Source: CAD feature listing. Evaluate the final solid. Frame: model axes, mm. Face numbers are marked on the shaded views. A direction names the side the tool comes from. Round coordinates to 2 decimals unless told otherwise and drop trailing zeros. Write each loop counter-clockwise with the first axis right and the second up, starting at its lowest first coordinate (ties: lowest second). Pieces come first, ordered by that corner, then holes.
Autodesk Inventor part; units mm, degrees
ref_plane "YZ Plane" through (0, 0, 0) normal (1, 0, 0) x (0, 1, 0)
ref_plane "XZ Plane" through (0, 0, 0) normal (0, 1, 0) x (-1, 0, 0)
ref_plane "XY Plane" through (0, 0, 0) normal (0, 0, 1) x (1, 0, 0)
sketch "Sketch1" plane through (0, 0, 0) normal (0, 0, 1) x (1, 0, 0)
  line L0 (17.9, -19.1) -> (17.9, 19.1)
  line L1 (15.9, 21.1) -> (-15.9, 21.1)
  line L2 (-17.9, 19.1) -> (-17.9, -19.1)
  line L3 (-15.9, -21.1) -> (-10.5924, -21.1)
  line L4 (17.9, -21.1) -> (-17.9, 21.1) construction
  line L5 (17.9, 21.1) -> (-17.9, -21.1) construction
  line L6 (-7.4, -17.4) -> (7.4, -17.4)
  line L7 (-7.4, -17.4) -> (-8.833, -20.051)
  line L8 (7.4, -17.4) -> (8.833, -20.051)
  line L9 (10.5924, -21.1) -> (15.9, -21.1)
  line L10 (-9.4, -21.1) -> (9.4, -21.1)
  arc A0 (-15.9, 21.1) -> (-17.9, 19.1) centre (-15.9, 19.1) ccw
  arc A1 (17.9, 19.1) -> (15.9, 21.1) centre (15.9, 19.1) ccw
  arc A2 (15.9, -21.1) -> (17.9, -19.1) centre (15.9, -19.1) ccw
  arc A3 (8.833, -20.051) -> (10.5924, -21.1) centre (10.5924, -19.1) ccw
  arc A4 (-10.5924, -21.1) -> (-8.833, -20.051) centre (-10.5924, -19.1) ccw
  arc A5 (-17.9, -19.1) -> (-15.9, -21.1) centre (-15.9, -19.1) ccw
  point P0 (0, 0)
  dimension "d0" = 35.8
  dimension "d1" = 42.2
  dimension "d2" = 38.5
  dimension "d3" = 10.5
  dimension "d4" = 10.5
  dimension "d5" = 8.5
  dimension "d6" = 8.5
  dimension "d7" = 2
extrude "Extrusion1" add sketch "Sketch1" along normal blind 1.8
sketch "Sketch2" plane through (0, 0, 1.8) normal (0, 0, 1) x (1, 0, 0)
  line L0 (-15.85, 15.1) -> (15.85, 15.1)
  line L1 (15.85, 15.1) -> (15.85, 17.6)
  line L2 (15.85, 17.6) -> (-15.85, 17.6)
  line L3 (-15.85, 17.6) -> (-15.85, 15.1)
  line L4 (-15.85, 15.1) -> (15.85, 17.6) construction
  line L5 (15.85, 15.1) -> (-15.85, 17.6) construction
  line L6 (15.9, 21.1) -> (-15.9, 21.1)
  point P0 (0, 0)
  point P1 (0, 16.35)
  point P2 (0, 16.35)
  point P3 (15.85, 16.35)
  point P4 (-15.85, 16.35)
  dimension "d10" = 2.5
  dimension "d11" = 6
  dimension "d12" = 31.7
extrude "Extrusion2" add sketch "Sketch2" along normal blind 1
fillet "Fillet1" radius 1 2 edges at (0, 17.6, 2.8) (0, 15.1, 2.8)
sketch "Sketch3" plane through (0, 0, 1.8) normal (0, 0, 1) x (1, 0, 0)
  line L0 (-12.9, 19.1) -> (12.9, 19.1)
  line L1 (13.9, 18.1) -> (13.9, -13.2)
  line L2 (12.9, -14.2) -> (-12.9, -14.2)
  line L3 (-13.9, -13.2) -> (-13.9, 18.1)
  line L4 (15.9, 21.1) -> (-15.9, 21.1)
  line L5 (-13.9, 2.9131) -> (-17.9, 2.9131)
  line L6 (-17.9, 19.1) -> (-17.9, -19.1)
  line L7 (13.9, 2.9131) -> (17.9, 2.9131)
  line L8 (17.9, -19.1) -> (17.9, 19.1)
  arc A0 (-12.9, 19.1) -> (-13.9, 18.1) centre (-12.9, 18.1) ccw
  arc A1 (13.9, 18.1) -> (12.9, 19.1) centre (12.9, 18.1) ccw
  arc A2 (12.9, -14.2) -> (13.9, -13.2) centre (12.9, -13.2) ccw
  arc A3 (-13.9, -13.2) -> (-12.9, -14.2) centre (-12.9, -13.2) ccw
  point P0 (0, 0)
  point P1 (13.9, -14.2)
  point P2 (13.9, 19.1)
  point P3 (-13.9, -14.2)
  dimension "d16" = 27.8
  dimension "d17" = 33.3
  dimension "d18" = 2
  dimension "d19" = 1
extrude "Extrusion3" add sketch "Sketch3" along normal blind 3.7
sketch "Sketch4" plane through (0, 0, 0) normal (0, 0, -1) x (-1, 0, 0)
  line L0 (-17.9, -19.1) -> (-17.9, 19.1)
  line L1 (17.9, 19.1) -> (17.9, -19.1)
  line L2 (-17.9, 6.6) -> (17.9, 6.6)
  line L3 (17.9, 6.6) -> (17.9, 4.1)
  line L4 (17.9, 4.1) -> (-17.9, 4.1)
  line L5 (-17.9, 4.1) -> (-17.9, 6.6)
  line L6 (-15.9, 21.1) -> (15.9, 21.1)
  point P0 (0, 0)
  dimension "d22" = 2.5
  dimension "d23" = 17
extrude "Extrusion4" add sketch "Sketch4" along normal blind 1
fillet "Fillet2" radius 1 2 edges at (0, 6.6, -1) (0, 4.1, -1)
sketch "Sketch5" plane through (0, 0, 0) normal (0, 0, -1) x (-1, 0, 0)
  line L0 (-14.8, 8.9) -> (14.8, 8.9)
  line L1 (15.8, 7.9) -> (15.8, -0.1)
  line L2 (14.8, -1.1) -> (-14.8, -1.1)
  line L3 (-15.8, -0.1) -> (-15.8, 7.9)
  line L4 (-15.9, 21.1) -> (15.9, 21.1)
  line L5 (-17.9, 6.6) -> (-17.9, 19.1)
  line L6 (17.9, 4.1) -> (17.9, -19.1)
  arc A0 (-15.8, -0.1) -> (-14.8, -1.1) centre (-14.8, -0.1) ccw
  arc A1 (-14.8, 8.9) -> (-15.8, 7.9) centre (-14.8, 7.9) ccw
  arc A2 (15.8, 7.9) -> (14.8, 8.9) centre (14.8, 7.9) ccw
  arc A3 (14.8, -1.1) -> (15.8, -0.1) centre (14.8, -0.1) ccw
  point P0 (0, 0)
  point P1 (0, 8.9)
  dimension "d27" = 22.2
  dimension "d28" = 2.1
  dimension "d29" = 10
  dimension "d30" = 2.1
  dimension "d31" = 1
extrude "Extrusion5" add sketch "Sketch5" along normal blind 26.3
sketch "Sketch6" plane through (0, 0, 0) normal (0, 0, -1) x (-1, 0, 0)
  line L0 (-5, 16.9799) -> (5, 16.9799)
  line L1 (5, 16.9799) -> (5, 8.9)
  line L2 (5, 8.9) -> (-5, 8.9)
  line L3 (-5, 8.9) -> (-5, 16.9799)
  line L4 (14.8, 8.9) -> (-14.8, 8.9)
  line L5 (5, 16.9799) -> (17.9, 16.9799)
  line L6 (17.9, 19.1) -> (17.9, 6.6)
  line L7 (-5, 16.9799) -> (-17.9, 16.9799)
  line L8 (-17.9, -19.1) -> (-17.9, 19.1)
  point P0 (0, 0)
  point P1 (-5, 12.94)
  dimension "d34" = 10
extrude "Extrusion6" cut sketch "Sketch6" against normal blind 4.5
sketch "Sketch7" plane through (-14.8, 8.9, -26.3) normal (0, 1, 0) x (1, 0, 0)
  line L0 (9.8, -30.8) -> (19.8, -30.8)
  line L1 (14.8, -30.8) -> (14.8, -11.8)
  line L2 (8.8, -11.8) -> (20.8, -11.8)
  line L3 (20.8, -11.8) -> (20.8, -10.8)
  line L4 (20.8, -10.8) -> (8.8, -10.8)
  line L5 (8.8, -10.8) -> (8.8, -11.8)
  line L6 (20.8, -11.8) -> (20.8, -26.3)
  line L7 (20.8, -26.3) -> (19.8, -26.3)
  line L8 (19.8, -26.3) -> (19.8, -11.8)
  line L9 (8.8, -11.8) -> (8.8, -26.3)
  line L10 (8.8, -26.3) -> (9.8, -26.3)
  line L11 (9.8, -26.3) -> (9.8, -11.8)
  point P0 (14.8, -26.3)
  dimension "d37" = 19
  dimension "d38" = 12
  dimension "d39" = 1
  dimension "d40" = 1
  dimension "d41" = 14.5
extrude "Extrusion7" add sketch "Sketch7" along normal blind 2
sketch "Sketch8" plane through (-14.8, 10.9, -26.3) normal (0, 1, 0) x (1, 0, 0)
  line L0 (9.8, -11.8) -> (19.8, -11.8)
  line L1 (20.8, -26.3) -> (20.8, -10.8)
  line L2 (19.8, -11.8) -> (20.8, -11.8)
  line L3 (20.8, -11.8) -> (20.8, -25.8)
  line L4 (20.8, -25.8) -> (19.8, -25.8)
  line L5 (19.8, -25.8) -> (19.8, -11.8)
  line L6 (9.8, -11.8) -> (9.8, -30.8)
  line L7 (8.8, -26.3) -> (8.8, -10.8)
  line L8 (9.8, -11.8) -> (8.8, -11.8)
  line L9 (8.8, -11.8) -> (8.8, -25.8)
  line L10 (8.8, -25.8) -> (9.8, -25.8)
  line L11 (9.8, -25.8) -> (9.8, -11.8)
  point P0 (14.8, -26.3)
  point P1 (9.8, -25.8)
  point P2 (9.8, -25.8)
extrude "Extrusion8" add sketch "Sketch8" along normal blind 2
sketch "Sketch9" plane through (5, 8.9, -14.5) normal (-1, 0, 0) x (0, 0, 1)
  line L0 (0, 2) -> (0, 4)
  line L1 (14, 0) -> (14, 4)
  line L2 (0, 4) -> (14, 4)
  line L3 (14, 4) -> (14, 2)
  line L4 (14, 2) -> (0, 2)
  line L5 (0, 2) -> (0, 4)
  point P0 (14.5, -8.9)
  point P1 (0, 2)
extrude "Extrusion9" add sketch "Sketch9" along normal blind 0.5
chamfer "Chamfer1" distance 2 angle 35 1 edges at (4.5, 12.9, -7.5) measured on face at (4.5, 11.5667, -5.1667)
mirror "Mirror1" about plane through (0, 0, 0) normal (1, 0, 0) of "Extrusion9", "Chamfer1"
sketch "Sketch10" plane through (0, 0, 4.5) normal (0, 0, -1) x (-1, 0, 0)
  line L0 (-4.5, 9.9) -> (4.5, 9.9)
  line L1 (5, 10.4) -> (5, 12.2)
  line L2 (4.5, 12.7) -> (-4.5, 12.7)
  line L3 (-5, 12.2) -> (-5, 10.4)
  line L4 (5, 8.9) -> (-5, 8.9)
  line L5 (-5, 8.9) -> (-5, 16.9799)
  arc A0 (-5, 10.4) -> (-4.5, 9.9) centre (-4.5, 10.4) ccw
  arc A1 (-4.5, 12.7) -> (-5, 12.2) centre (-4.5, 12.2) ccw
  arc A2 (5, 12.2) -> (4.5, 12.7) centre (4.5, 12.2) ccw
  arc A3 (4.5, 9.9) -> (5, 10.4) centre (4.5, 10.4) ccw
  point P0 (0, 0)
  point P1 (-5, 11.3)
  dimension "d51" = 1
  dimension "d52" = 10
  dimension "d53" = 0.5
  dimension "d54" = 2.8
extrude "Extrusion10" cut sketch "Sketch10" against normal blind 2
properties part number "PS2 USB C PD Mount"
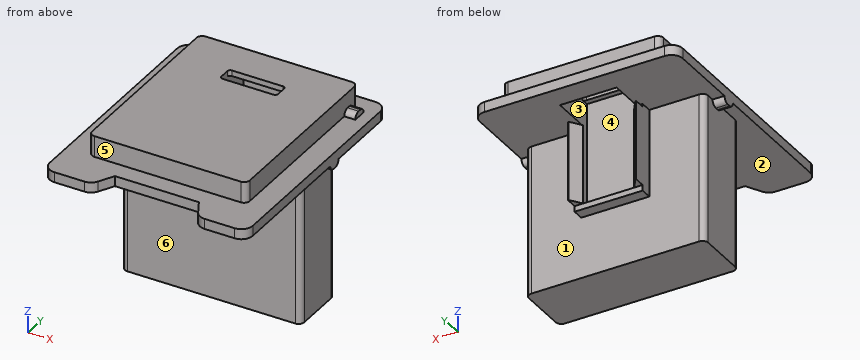
1) Section query A-A on x = -1.5. Return the cut outline in (y, z).
Taken from the geometry:
outline: (-17.4, 0) - (-1.1, 0) - (-1.1, -26.3) - (8.9, -26.3) - (8.9, -15.5) - (10.9, -15.5) - (10.9, -14.5) - (8.9, -14.5) - (8.9, 4.5) - (9.9, 4.5) - (9.9, 5.5) - (-14.2, 5.5) - (-14.2, 1.8) - (-17.4, 1.8) - close; (12.7, 4.5) - (16.98, 4.5) - (16.98, 0) - (21.1, 0) - (21.1, 1.8) - (19.1, 1.8) - (19.1, 5.5) - (12.7, 5.5) - close
2) Contact query for flat-ended pins moving along their axis: P1, Ø1.5, axis at x = 6, y = -6, coming from the -Z side; P2, Ø0.6, axis at x = 1.5, y = 10, coming from the -Z side; P3, Ø3, axis at x = -1.5, z = -9.5, coming from the +Y side; P4, Ø3, axis at x = -0.5, z = 3, coming from the +Y side. Output: stop coordinate, or through.
Taken from the geometry:
P1: stops at z = 0
P2: stops at z = -15.5
P3: stops at y = 8.9
P4: stops at y = 21.1
3) Section query C-C on z = -20. Return the cut outline in (x, y).
Taken from the geometry:
outline: (-15.8, -0.1) arc R1 ccw to (-14.8, -1.1) - (14.8, -1.1) arc R1 ccw to (15.8, -0.1) - (15.8, 7.9) arc R1 ccw to (14.8, 8.9) - (-14.8, 8.9) arc R1 ccw to (-15.8, 7.9) - close
4) Reachability of the marked faces 4, 5 and 6 from +Z, -Z, +X, -X, +Y, -Y: full face, straight path, thin tool, end or side. Return the list, or none.
Taken from the geometry:
face 4: none
face 5: +Z, +X, -X, -Y
face 6: -Z, +X, -X, -Y
5) Material intervals for line 1 (Z direction, x = 15, y = 9.5); line 2 (Y direction, x = 9.5, z = -3); line 3 (Z direction, x = -13, y = 9.5), sorted ascending.
Taken from the geometry:
line 1: z = 0 to 1.8
line 2: y = -1.1 to 8.9
line 3: z = 0 to 5.5
6) Section query D-D on x = -8. Return the cut outline in (y, z).
Taken from the geometry:
outline: (-18.51, 0) - (-1.1, 0) - (-1.1, -26.3) - (8.9, -26.3) - (8.9, 0) - (21.1, 0) - (21.1, 1.8) - (19.1, 1.8) - (19.1, 5.5) - (-14.2, 5.5) - (-14.2, 1.8) - (-18.51, 1.8) - close
7) Pull-direction query (Z, two-part tool) for the marked faces 1, 2 and 3; classes: released by +Z, released by -Z, zero draft, split by the parting line, or undercut.
Taken from the geometry:
face 1: zero draft
face 2: released by -Z
face 3: undercut
8) Section query B-B on y = -10.5. Return the cut outline in (x, z).
Taken from the geometry:
outline: (-17.9, 0) - (17.9, 0) - (17.9, 1.8) - (13.9, 1.8) - (13.9, 5.5) - (-13.9, 5.5) - (-13.9, 1.8) - (-17.9, 1.8) - close
